Model file for the job. Use its own axes, mm. A direction names the side the tool comes from. Round coordinates to 2 decimals unless told otherwise and drop trailing zeros. Write each loop counter-clockwise with the first axis right and the second up, starting at its lowest first coordinate (ties: lowest second). Pieces come first, ordered by that corner, then holes. Notation, with made-up numbers: (-27.5, 1.5) - (-17.5, 1.5) arc R37 ccw to (-17.5, 39.5) - close; hole circle Ø5 at (-14.75, 47). An arc over 180 degrees is marked (long way). One line per item, written item: value.
from build123d import *

# Parameters (mm, degrees)
SKETCH_1_R          = 14.25
SKETCH_1_R_2        = 12.4
EXTRUDE_1_DEPTH     = 13.5
EXTRUDE_START       = 2
SKETCH_2_R          = 14.25
SKETCH_2_R_2        = 4.5
SKETCH_2_R_3        = 1.5
EXTRUDE_2_DEPTH     = 2
SKETCH_4_W          = 16.5
SKETCH_4_H          = 7.711801842
CUT_EXTRUDE_2_DEPTH = 19


with BuildPart() as part:
    # 草图1 → 凸台-拉伸1 (new body)
    with BuildSketch(Plane.XY):
        Circle(SKETCH_1_R)
        Circle(SKETCH_1_R_2, mode=Mode.SUBTRACT)
    extrude(amount=EXTRUDE_1_DEPTH)

    # 草图2 → 凸台-拉伸2 (add)
    with BuildSketch(Plane(origin=(0, 0, 0), x_dir=(-1, 0, 0), z_dir=(0, 0, -1)).offset(EXTRUDE_START)):
        Circle(SKETCH_2_R)
        Circle(SKETCH_2_R_2, mode=Mode.SUBTRACT)
        with Locations((-10, 0)):
            Circle(SKETCH_2_R_3, mode=Mode.SUBTRACT)
    extrude(amount=-EXTRUDE_2_DEPTH)

    # 草图4 → 切除-拉伸2 (cut)
    with BuildSketch(Plane.XY.offset(13.5)):
        with Locations((0, -12.4)):
            Rectangle(SKETCH_4_W, SKETCH_4_H)
    extrude(amount=-CUT_EXTRUDE_2_DEPTH, mode=Mode.SUBTRACT)


solid = part.part
1. Mould opens along X. For faces 1 (the face through (-8.25, -10, 6)), 2 (the face through (-3, 4, -2)), 3 (the face through (-0.5, 14.24, 5.64)) say: released by +X, released by -X, zero draft, split by the parting line, or undercut.
Report:
face 1: undercut
face 2: zero draft
face 3: split by the parting line
2. Band-saw the part on B-B on x = 0. Write the cut outline in (y, z), plus the area to 3 significant figures.
Report:
outline: (-8.54, -2) - (-4.5, -2) - (-4.5, 0) - (-8.54, 0) - close; (4.5, -2) - (14.25, -2) - (14.25, 13.5) - (12.4, 13.5) - (12.4, 0) - (4.5, 0) - close
area: 52.6 mm²
3. Band-saw the part on A-A on y = 0. Write the cut outline in (x, z).
Report:
outline: (-14.25, -2) - (-4.5, -2) - (-4.5, 0) - (-12.4, 0) - (-12.4, 13.5) - (-14.25, 13.5) - close; (4.5, -2) - (8.5, -2) - (8.5, 0) - (4.5, 0) - close; (11.5, -2) - (14.25, -2) - (14.25, 13.5) - (12.4, 13.5) - (12.4, 0) - (11.5, 0) - close
4. Wall check: probe 1 along Y at (x, z) = (0, -0.9); probe 2 along X at (y, z) = (-0.25, 3.25); probe 3 along Z at (x, y) = (-6.5, -4). Give the ranges that are in metal, low to high. Write a range as [from, to].
Report:
probe 1: [-8.54, -4.5], [4.5, 14.25]
probe 2: [-14.25, -12.4], [12.4, 14.25]
probe 3: [-2, 0]
5. Band-saw the part on C-C on z = 7.5. Write the cut outline in (x, y).
Report:
outline: (-8.25, -11.62) - (-8.25, -9.26) arc R12.4 cw (long way) to (8.25, -9.26) - (8.25, -11.62) arc R14.25 ccw (long way) to start
6. Drop flat-ended pins along their axis: pin 1 (1.5 mm diameter, centred on y = -5.5, z = 11.5, fed in from -X) (3 decimals); pin 2 (4 mm diameter, centred on x = 10, y = 0, fed in from +Z); pin 3 (1 mm diameter, centred on x = 9.5, z = 9.5, fed in from -Y). Give the stop position or say it passes through.
Report:
pin 1: x = -13.435
pin 2: z = 0
pin 3: y = -11.05
7. Tool access for faces 4 (the face through (-4, 12, 13.5)), 5 (the face through (-3, 4, 0)), 6 (the face through (8.25, -10, 6)): list every direction of +Z, -Z, +X, -X, +Y, -Y with a clear straight run to the whole face (end or side of a thin tool).
Report:
face 4: +Z, +X, -X, +Y, -Y
face 5: +Z
face 6: +Z, -Z, -Y
8. Band-saw the part on D-D on x = 10. Write the cut outline in (y, z).
Report:
outline: (-10.15, -2) - (-1.5, -2) - (-1.5, 0) - (-7.33, 0) - (-7.33, 13.5) - (-10.15, 13.5) - close; (1.5, -2) - (10.15, -2) - (10.15, 13.5) - (7.33, 13.5) - (7.33, 0) - (1.5, 0) - close
